from build123d import *

# Parameters (mm, degrees)
F0_W     = 200
F0_H     = 270
F1_DEPTH = 10
F2_W     = 10
F2_H     = 130
F3_DEPTH = 310
F5_D     = 14


with BuildPart() as f1:
    # F0 (on Top) → F1 (new body)
    with BuildSketch(Plane.XY):
        with Locations((100, 135)):
            Rectangle(F0_W, F0_H)
    extrude(amount=F1_DEPTH)

    # F2 (on face) → F3 (join)
    with BuildSketch(Plane.XY.offset(10)):
        with Locations((139, 200)):
            Rectangle(F2_W, F2_H)
    extrude(amount=F3_DEPTH)

    # F5 (through all)
    with Locations(Plane.YZ.offset(144)):
        with Locations((150, 290), (250, 290), (250, 170), (150, 170), (150, 50), (250, 50)):
            Hole(F5_D / 2)


solid = f1.part
For this review, take the finished solid that the model builds, in its own axes (mm). A direction names the side the tool comes from. Give positions to 0.01 mm unless a question says otherwise; leave off trailing zeros. Loops run counter-clockwise (first coordinate to the right, second up) from the corner with the lowest first, then second, coordinate; pieces in that order, holes last. Notation, with made-up numbers: M -19.75,38 L 30.25,38 A14 ccw 30.25,42 Z; hole C -14.5,-39 d5. An arc over 180 degrees is marked long. Answer as a JSON object with one key per item and string values. Group by question number.
Q1. Tool access review of faces 5 (the flat face through (200, 133, 5)), 6 (the flat face through (134, 199, 163)), 7 (the flat face through (139, 135, 163)), 8 (the flat face through (139, 265, 163)), 9 (the flat face through (144, 199, 163)): name each direction out of +Z, -Z, +X, -X, +Y, -Y from which nothing blocks a thin tool from reaching the whole face with its end or side.
Q2. Add section A-A on z = 50. Give the boundary of the cut face in (x, y).
Q3. For probe 1 along Z at (x, y) = (138, 250); probe 2 along Y at (x, z) = (139.25, 290); probe 3 along X at (y, z) = (202.5, 242), list the stretches that pass through material, from the lowest coordinate up. Write a range as [from, to].
Q4. Add section C-C on x = 108.5. Give the boundary of the cut face in (y, z).
Q5. Add section B-B on y = 150. Give the boundary of the cut face in (x, z), and give its area (3 significant figures).
Q6. Insertion check: P1, Ø22.5, axis at y = 250, z = 170, coming from the +X side; P2, Ø1, axis at x = 136, z = 130, coming from the +Y side; P3, Ø3, axis at x = 138, z = 165.5, coming from the -Y side. Each pin has a flat end and moves straight along its axis. Give the tip position at first contact, or say it passes through.
Q7. Add section D-D on y = 48. Give the boundary of the cut face in (x, z).
Q8. Mouldability with a two-part tool opening along Y and no side actions: class faces 1 (the cylindrical face through (138.93, 243.534, 287.319)), 2 (the flat face through (99, 270, 5)), 3 (the cylindrical face through (138.93, 151.517, 283.166)), 4 (the flat face through (0, 133, 5)) as +Y half, -Y half, draft (parallel to the pull), parting line (faces both ways), or undercut.
Checked values:
{
 "1": {"face 5": "+Z, -Z, +X, +Y, -Y", "face 6": "+Z, -X, +Y, -Y", "face 7": "+Z, +X, -X, -Y", "face 8": "+Z, +X, -X, +Y", "face 9": "+Z, +X, +Y, -Y"},
 "2": {"outline": "M 134,135 L 144,135 L 144,143 L 134,143 Z; M 134,157 L 144,157 L 144,243 L 134,243 Z; M 134,257 L 144,257 L 144,265 L 134,265 Z"},
 "3": {"probe 1": "[0, 43], [57, 163], [177, 283], [297, 320]", "probe 2": "[135, 143], [157, 243], [257, 265]", "probe 3": "[134, 144]"},
 "4": {"outline": "M 0,0 L 270,0 L 270,10 L 0,10 Z"},
 "5": {"outline": "M 0,0 L 200,0 L 200,10 L 144,10 L 144,43 L 134,43 L 134,10 L 0,10 Z; M 134,57 L 144,57 L 144,163 L 134,163 Z; M 134,177 L 144,177 L 144,283 L 134,283 Z; M 134,297 L 144,297 L 144,320 L 134,320 Z", "area": "4,680 mm²"},
 "6": {"P1": "x = 144", "P2": "y = 265", "P3": "y = 135"},
 "7": {"outline": "M 0,0 L 200,0 L 200,10 L 0,10 Z"},
 "8": {"face 1": "undercut", "face 2": "+Y half", "face 3": "undercut", "face 4": "draft"}
}
